```python
from build123d import *

# Parameters (mm, degrees)
SKETCH1_W           = 25
SKETCH1_H           = 62
BOSS_EXTRUDE1_DEPTH = 10


with BuildPart() as part:
    # Sketch1 → Boss-Extrude1 (new body)
    with BuildSketch(Plane(origin=(0, 0, 0), x_dir=(0, 0, -1), z_dir=(1, 0, 0))):
        Rectangle(SKETCH1_W, SKETCH1_H)
    extrude(amount=BOSS_EXTRUDE1_DEPTH)

    # Sketch2 → Cut-Revolve1 (revolve, cut)
    with BuildSketch(Plane(origin=(0, 26, 0), x_dir=(-1, 0, 0), z_dir=(0, 1, 0))):
        Polygon((0, -8), (0, -10.5), (-0.433, -10.067), (-9.567, -10.067), (-10, -10.5), (-10, -8), align=None)
    revolve(axis=Axis((10, 26, -8), (-1, 0, 0)), mode=Mode.SUBTRACT)

    # Sketch3 → Cut-Revolve2 (revolve, cut)
    with BuildSketch(Plane(origin=(0, -26, 0), x_dir=(-1, 0, 0), z_dir=(0, 1, 0))):
        Polygon((0, -8), (0, -10.5), (-0.433, -10.067), (-9.567, -10.067), (-10, -10.5), (-10, -8), align=None)
    revolve(axis=Axis((10, -26, -8), (-1, 0, 0)), mode=Mode.SUBTRACT)

    # Sketch4 → Cut-Revolve3 (revolve, cut)
    with BuildSketch(Plane(origin=(0, -26, 0), x_dir=(-1, 0, 0), z_dir=(0, 1, 0))):
        Polygon((0, 8), (0, 5.5), (-0.433, 5.933), (-9.567, 5.933), (-10, 5.5), (-10, 8), align=None)
    revolve(axis=Axis((10, -26, 8), (-1, 0, 0)), mode=Mode.SUBTRACT)

    # Sketch5 → Cut-Revolve4 (revolve, cut)
    with BuildSketch(Plane(origin=(0, 26, 0), x_dir=(-1, 0, 0), z_dir=(0, 1, 0))):
        Polygon((0, 8), (0, 5.5), (-0.433, 5.933), (-9.567, 5.933), (-10, 5.5), (-10, 8), align=None)
    revolve(axis=Axis((10, 26, 8), (-1, 0, 0)), mode=Mode.SUBTRACT)

    # Sketch6 → Cut-Revolve5 (revolve, cut)
    with BuildSketch(Plane(origin=(0, 23, 0), x_dir=(-1, 0, 0), z_dir=(0, 1, 0))):
        Polygon((0, 0), (0, -3.8), (-5.555555556, -3.8), (-5.555555556, -3.5), (-2.055555556, -3.5), (-1.555555556, -3), (-1.555555556, -1.5), (-4.155555556, -1.5), (-5.021580959, 0), align=None)
    revolve(axis=Axis((5.021580959, 23, 0), (-1, 0, 0)), mode=Mode.SUBTRACT)

    # Sketch7 → Cut-Revolve6 (revolve, cut)
    with BuildSketch(Plane(origin=(0, 0, 0), x_dir=(-1, 0, 0), z_dir=(0, 1, 0))):
        Polygon((0, 0), (0, -3.8), (-5.555555556, -3.8), (-5.555555556, -3.5), (-2.055555556, -3.5), (-1.555555556, -3), (-1.555555556, -1.5), (-4.155555556, -1.5), (-5.021580959, 0), align=None)
    revolve(axis=Axis((5.021580959, 0, 0), (-1, 0, 0)), mode=Mode.SUBTRACT)

    # Sketch8 → Cut-Revolve7 (revolve, cut)
    with BuildSketch(Plane(origin=(0, -23, 0), x_dir=(-1, 0, 0), z_dir=(0, 1, 0))):
        Polygon((0, 0), (0, -3.8), (-5.555555556, -3.8), (-5.555555556, -3.5), (-2.055555556, -3.5), (-1.555555556, -3), (-1.555555556, -1.5), (-4.155555556, -1.5), (-5.021580959, 0), align=None)
    revolve(axis=Axis((5.021580959, -23, 0), (-1, 0, 0)), mode=Mode.SUBTRACT)

    # Sketch9 → Revolve1 (revolve)
    with BuildSketch(Plane(origin=(0, 0, 0), x_dir=(-1, 0, 0), z_dir=(0, 1, 0))):
        Polygon((-10, 0), (-10, -4), (-61.6, -4), (-62, -3.6), (-62, 0), align=None)
    revolve(axis=Axis((62, 0, 0), (-1, 0, 0)))

    # Sketch10 → Revolve2 (revolve)
    with BuildSketch(Plane(origin=(0, -23, 0), x_dir=(-1, 0, 0), z_dir=(0, 1, 0))):
        Polygon((-10, 0), (-10, -4), (-113.6, -4), (-114, -3.6), (-114, 0), align=None)
    revolve(axis=Axis((114, -23, 0), (-1, 0, 0)))

    # Sketch11 → Revolve3 (revolve)
    with BuildSketch(Plane(origin=(0, 23, 0), x_dir=(-1, 0, 0), z_dir=(0, 1, 0))):
        Polygon((-10, 0), (-10, -4), (-113.6, -4), (-114, -3.6), (-114, 0), align=None)
    revolve(axis=Axis((114, 23, 0), (-1, 0, 0)))


solid = part.part
```
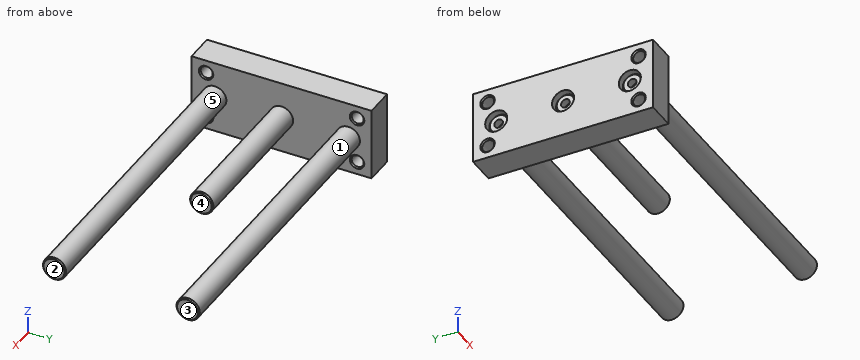
Could you check a few things on this model? Use its own coordinates, in mm. Face numbers are marked on the shaded views. A direction names the side the tool comes from. Round coordinates to 2 decimals unless told otherwise and drop trailing zeros. Write each loop counter-clockwise with the first axis right and the second up, starting at its lowest first coordinate (ties: lowest second). Pieces come first, ordered by that corner, then holes.
(1) For pin 1 (2.5 mm diameter, centred on y = 0, z = 0, fed in from -X); pin 2 (6 mm diameter, centred on y = 0, z = 0, fed in from +X); pin 3 (2.5 mm diameter, centred on y = -24.5, z = 0, fed in from -X), each with a flat end and sliding along its axis, tell me the tip position at first contact or that it passes through.
Findings below:
pin 1: stops at x = 4.3
pin 2: stops at x = 62
pin 3: stops at x = 1.56
(2) Suppose I cut it at C-C on y = -9. Write out the boundary of the cut face in (x, z).
Findings below:
outline: (0, -12.5) - (10, -12.5) - (10, 12.5) - (0, 12.5) - close
(3) Suppose I cut it at B-B on x = 17.5. Write out the boundary of the cut face in (y, z).
Findings below:
outline: circle Ø8 at (-23, 0); circle Ø8 at (0, 0); circle Ø8 at (23, 0)
(4) Suppose I cut it at D-D on z = 7.5. State how many separate pieces and enclosed holes the cut face has, and give its area (3 significant figures).
Findings below:
separate pieces: 3
enclosed holes: 0
area: 539 mm2
(5) If I drill on probe 1 along Z at (x, y) = (2.7, 0); probe 2 along Y at (x, z) = (4.75, 8); probe 3 along Z at (x, y) = (2.5, 26), over which ranges is the centre line in solid material (lowest first)?
Findings below:
probe 1: z = -12.5 to -3.8, -3.5 to -1.5, 1.5 to 3.5, 3.8 to 12.5
probe 2: y = -31 to -28.07, -23.93 to 23.93, 28.07 to 31
probe 3: z = -12.5 to -10.07, -5.93 to -2.33, -1.8 to 1.8, 2.33 to 5.93, 10.07 to 12.5
(6) Suppose I cut it at A-A on z = -8. Write out the boundary of the cut face in (x, y).
Findings below:
outline: (0, -31) - (10, -31) - (10, -28.5) - (9.57, -28.07) - (0.43, -28.07) - (0, -28.5) - close; (0, -23.5) - (0.43, -23.93) - (9.57, -23.93) - (10, -23.5) - (10, 23.5) - (9.57, 23.93) - (0.43, 23.93) - (0, 23.5) - close; (0, 28.5) - (0.43, 28.07) - (9.57, 28.07) - (10, 28.5) - (10, 31) - (0, 31) - close
(7) Thinking about a two-plate mould opening in Y: for the marked faces 1 and 2, which applies, +Y half, -Y half, draft (parallel to the pull), parting line (faces both ways), or undercut?
Findings below:
face 1: undercut
face 2: draft
(8) Which directions (+Z, -Z, +X, -X, +Y, -Y) give clear straight access to the entire face, cutting with the end or side of a thin tool? Please do the marked faces 3, 4 and 5.
Findings below:
face 3: +Z, -Z, +X, +Y, -Y
face 4: +Z, -Z, +X
face 5: +X
